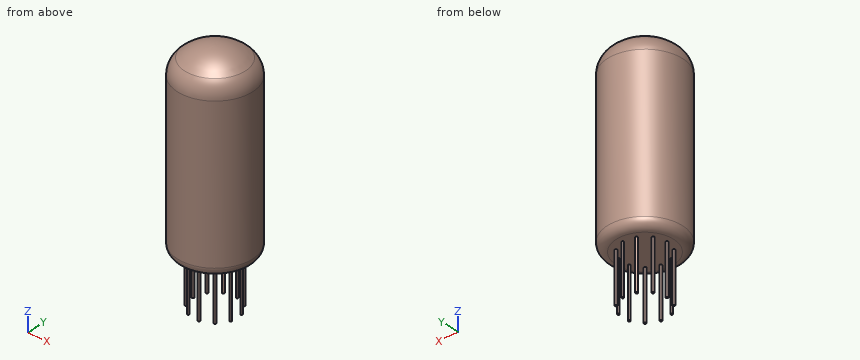
from build123d import *

# Parameters (mm, degrees)
F2_R     = 2.1
F3_R     = 0.25
F4_DEPTH = 12


with BuildPart() as f1:
    # F0 (on Right) → F1 (revolve)
    with BuildSketch(Plane.YZ):
        with BuildLine():
            Line((-8.95, 38.106404), (-8.95, 0))
            Line((-8.95, 0), (0, 0))
            Line((0, 0), (0, 44.565391))
            ThreePointArc((0, 44.565391), (-3.850647, 43.879973), (-7.218062, 41.890551))
            ThreePointArc((-7.218062, 41.890551), (-8.496444, 40.187232), (-8.95, 38.106404))
        make_face()
    revolve(axis=Axis((0, 0, 22.282695), (0, 0, 1)))

    # F2
    f2_edges = [f1.edges().sort_by_distance(p)[0] for p in [
        (0, 8.95, 0),
    ]]
    fillet(f2_edges, radius=F2_R)

    # F3 (on face) → F4 (join)
    with BuildSketch(Plane(origin=(0, 0, 0), x_dir=(1, 0, 0), z_dir=(0, 0, -1))):
        with Locations((-5.35, 0)):
            Circle(F3_R)
        with Locations((-4.500706, -2.892428)):
            Circle(F3_R)
        with Locations((-2.22247, -4.866531)):
            Circle(F3_R)
        with Locations((0.761384, -5.295545)):
            Circle(F3_R)
        with Locations((3.503505, -4.04326)):
            Circle(F3_R)
        with Locations((5.133287, -1.507269)):
            Circle(F3_R)
        with Locations((5.133287, 1.507269)):
            Circle(F3_R)
        with Locations((3.503505, 4.04326)):
            Circle(F3_R)
        with Locations((0.761384, 5.295545)):
            Circle(F3_R)
        with Locations((-2.22247, 4.866531)):
            Circle(F3_R)
        with Locations((-4.500706, 2.892428)):
            Circle(F3_R)
    extrude(amount=F4_DEPTH)


solid = f1.part
Design review of the part built by this model. Coordinates are the model's own, in mm. Round coordinates to 2 decimals unless told otherwise and drop trailing zeros.
1) Consider section A-A (z = -1). Count the separate pieces of the cut face and the enclosed holes in it, plus the area to 3 significant figures.
The answers:
separate pieces: 11
enclosed holes: 0
area: 2.16 mm2
2) Clearance check with flat-ended pins moving along their axes: pin 1 Ø4 at (x, z) = (1, -2.5) entering from +Y; pin 2 Ø1 at (x, z) = (7, -6) entering from +Y; pin 3 Ø3 at (x, y) = (-2, -2.5) entering from +Z; pin 4 Ø1.5 at (x, y) = (-3.5, 5.5) entering from +Z. State where each tip first meets the part, or that it passes through.
The answers:
pin 1: stops at y = 5.55
pin 2: passes through
pin 3: stops at z = 44.44
pin 4: stops at z = 42.95
3) For L1, parallel to X at y = -5.75, z = 12.5; L2, parallel to X at y = -7.5, z = 1; L3, parallel to Y at x = -2, z = 21, list the stretches that pass through material, from the lowest coordinate up.
The answers:
L1: x = -6.86 to 6.86
L2: x = -4.29 to 4.29
L3: y = -8.72 to 8.72
